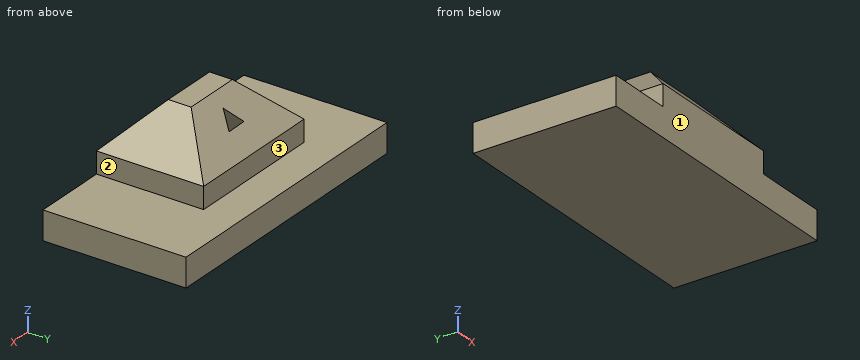
```python
from build123d import *

# Parameters (mm, degrees)
F0_W      = 1016
F0_H      = 508
F1_DEPTH  = 101.6
F4_W      = 237.9516797066
F4_H      = 381
F4_W_2    = 270.0483202934
F5_DEPTH  = 76.2
F5_FACE_W = 508
F5_FACE_H = 381
F6_DEPTH  = 149.86
F6_TAPER  = 45
F8_DEPTH  = 76.2


# Not quite as in the source:
# - the program builds the solid bodies; features that only make, move or delete a surface that nothing else refers to are left out


with BuildPart() as f1:
    # F0 (on Top) → F1 (new body)
    with BuildSketch(Plane.XY):
        Rectangle(F0_W, F0_H)
    extrude(amount=F1_DEPTH)

    # F4 (on face) → F5 (join)
    with BuildSketch(Plane.XY.offset(101.6)):
        with Locations((118.9758398533, -63.5)):
            Rectangle(F4_W, F4_H)
        with Locations((-135.0241601467, -63.5)):
            Rectangle(F4_W_2, F4_H)
    extrude(amount=F5_DEPTH)

    # F5_face (on face) → F6 (join, symmetric)
    with BuildSketch(Plane(origin=(-16.0483202934, -63.5, 177.8), x_dir=(1, 0, 0), z_dir=(0, 0, 1))):
        Rectangle(F5_FACE_W, F5_FACE_H)
    extrude(amount=F6_DEPTH, both=True, taper=F6_TAPER)

    # F7 (on face) → F8 (cut)
    with BuildSketch(Plane(origin=(0, 152.4, 152.4), x_dir=(-1, 0, 0), z_dir=(0, 0.7071067812, 0.7071067812))):
        Polygon((-18.2156057455, 126.8785575445), (57.9806947666, 127.6294159035), (19.232282097, 193.2419186418), align=None)
    extrude(amount=-F8_DEPTH, mode=Mode.SUBTRACT)


solid = f1.part
```
Part model, mm, in its own coordinate system. Face numbers are marked on the shaded views. A direction names the side the tool comes from. Round coordinates to 2 decimals unless told otherwise and drop trailing zeros. Write each loop counter-clockwise with the first axis right and the second up, starting at its lowest first coordinate (ties: lowest second). Pieces come first, ordered by that corner, then holes.
Item 1: Cut at A-A, the plane z = 205.5. Give the cut face in (x, y), plus the area to 3 significant figures.
Results:
outline: (-242.35, -226.3) - (210.25, -226.3) - (210.25, 99.3) - (-242.35, 99.3) - close; hole (-57.98, 25) - (-44, -8.46) - (4.44, -8.46) - (18.22, 26.07) - close
area: 145,000 mm2
Item 2: Which spindle directions (+Z, -Z, +X, -X, +Y, -Y) get a long thin tool onto all of the face, cutting with end or side? Do the marked faces 1, 2 and 3. Say none if no direction does.
Results:
face 1: +Z, -Z, +X, -X, -Y
face 2: +Z, +X, +Y, -Y
face 3: +Z, +X, -X, +Y
Item 3: Drop a flat-ended pin along its axis: pin 1 Ø1.5 at (x, z) = (16.5, 162) entering from +Y. Give the stop position or say it passes through.
Results:
pin 1: stops at y = 127
Item 4: Cut at C-C, the plane x = -195.5. Give the cut face in (y, z).
Results:
outline: (-254, 0) - (254, 0) - (254, 101.6) - (127, 101.6) - (127, 177.8) - (52.45, 252.35) - (-179.45, 252.35) - (-254, 177.8) - close
Item 5: Probe L1, parallel to Y at x = 48, z = 168; L2, parallel to Z at x = -336, y = -232.5; L3, parallel to Y at x = -160, z = 178. List the from-to ranges inside material, lowest first.
Results:
L1: y = -254 to 127
L2: z = 0 to 101.6
L3: y = -253.8 to 126.8
Item 6: Cut at B-B, the plane y = -67.5. Give the cut face in (x, z).
Results:
outline: (-508, 0) - (508, 0) - (508, 101.6) - (237.95, 101.6) - (237.95, 177.8) - (88.09, 327.66) - (-120.19, 327.66) - (-270.05, 177.8) - (-270.05, 101.6) - (-508, 101.6) - close
Item 7: Cut at D-D, the plane z = 275. Give the cut face in (x, y), plus the area to 3 significant figures.
Results:
outline: (-172.85, -156.8) - (140.75, -156.8) - (140.75, 29.8) - (-8.03, 29.8) - (-19.23, 1.71) - (-30.96, 29.8) - (-172.85, 29.8) - close
area: 58,200 mm2
